from build123d import *

# Parameters (mm, degrees)
BOSS_EXTRUDE1_OUTLINE_R = 16
BOSS_EXTRUDE1_DEPTH     = 10
SKETCH2_R               = 3.025
CUT_EXTRUDE1_DEPTH      = 25.738633754
CUT_EXTRUDE2_START      = -7.5
SKETCH3_R               = 16
SKETCH3_R_2             = 6.025
CUT_EXTRUDE2_DEPTH      = 7.5
SKETCH4_R               = 1.25
CUT_EXTRUDE3_DEPTH      = 10
CUT_EXTRUDE4_DEPTH      = 10
BOSS_EXTRUDE2_START     = -2.5
BOSS_EXTRUDE2_DEPTH     = 2.5
BOSS_EXTRUDE3_START     = 2.5
SKETCH9_R               = 3.025
BOSS_EXTRUDE3_DEPTH     = 2.5
SKETCH10_R              = 5.025
CUT_EXTRUDE5_DEPTH      = 2


# Read off the part's stored shape, not the designer's step: Boss-Extrude1, Boss-Extrude2
with BuildPart() as part:
    # Boss-Extrude1 outline → Boss-Extrude1 (new body)
    with BuildSketch(Plane(origin=(0, 0, 0), x_dir=(1, 0, 0), z_dir=(0, 1, 0))):
        Circle(BOSS_EXTRUDE1_OUTLINE_R)
    extrude(amount=BOSS_EXTRUDE1_DEPTH)

    # Sketch2 → Cut-Extrude1 (cut, through all)
    with BuildSketch(Plane(origin=(0, 10, 0), x_dir=(1, 0, 0), z_dir=(0, 1, 0))):
        with Locations(Location((0, 0, 0), (0, 0, 270))):
            Circle(SKETCH2_R)
    extrude(amount=-CUT_EXTRUDE1_DEPTH, mode=Mode.SUBTRACT)

    # Sketch3 → Cut-Extrude2 (cut)
    with BuildSketch(Plane(origin=(0, 10, 0), x_dir=(1, 0, 0), z_dir=(0, 1, 0)).offset(CUT_EXTRUDE2_START)):
        with Locations(Location((0, 0, 0), (0, 0, 270))):
            Circle(SKETCH3_R)
        with Locations(Location((0, 0, 0), (0, 0, 270))):
            Circle(SKETCH3_R_2, mode=Mode.SUBTRACT)
    extrude(amount=CUT_EXTRUDE2_DEPTH, mode=Mode.SUBTRACT)

    # Sketch4 → Cut-Extrude3 (cut)
    with BuildSketch(Plane.XY):
        with Locations((0, 6.5)):
            Circle(SKETCH4_R)
    extrude(amount=-CUT_EXTRUDE3_DEPTH, mode=Mode.SUBTRACT)

    # Sketch5 → Cut-Extrude4 (cut)
    with BuildSketch(Plane(origin=(0, 0, 0), x_dir=(-1, 0, 0), z_dir=(0, -1, 0))):
        with BuildLine():
            Line((0.210340042, 14.04358534), (0.548392997, 8.04358534))
            ThreePointArc((0.548392997, 8.04358534), (-0.393770609, 6.988915846), (-1.448440102, 7.931079452))
            Line((-1.448440102, 7.931079452), (-1.786493057, 13.931079452))
            ThreePointArc((-1.786493057, 13.931079452), (-0.844329452, 14.985748945), (0.210340042, 14.04358534))
        make_face()
        with BuildLine():
            Line((13.931079452, 1.786493057), (7.931079452, 1.448440102))
            ThreePointArc((7.931079452, 1.448440102), (6.988915846, 0.393770609), (8.04358534, -0.548392997))
            Line((8.04358534, -0.548392997), (14.04358534, -0.210340042))
            ThreePointArc((14.04358534, -0.210340042), (14.985748945, 0.844329452), (13.931079452, 1.786493057))
        make_face()
        with BuildLine():
            Line((1.786493057, -13.931079452), (1.448440102, -7.931079452))
            ThreePointArc((1.448440102, -7.931079452), (0.393770609, -6.988915846), (-0.548392997, -8.04358534))
            Line((-0.548392997, -8.04358534), (-0.210340042, -14.04358534))
            ThreePointArc((-0.210340042, -14.04358534), (0.844329452, -14.985748945), (1.786493057, -13.931079452))
        make_face()
        with BuildLine():
            Line((-13.931079452, -1.786493057), (-7.931079452, -1.448440102))
            ThreePointArc((-7.931079452, -1.448440102), (-6.988915846, -0.393770609), (-8.04358534, 0.548392997))
            Line((-8.04358534, 0.548392997), (-14.04358534, 0.210340042))
            ThreePointArc((-14.04358534, 0.210340042), (-14.985748945, -0.844329452), (-13.931079452, -1.786493057))
        make_face()
    extrude(amount=-CUT_EXTRUDE4_DEPTH, mode=Mode.SUBTRACT)

    # Boss-Extrude2 outline → Boss-Extrude2 (add)
    with BuildSketch(Plane.XZ.offset(BOSS_EXTRUDE2_START)):
        with BuildLine():
            Line((-4.70856839, 45.405985014), (-4.262641267, 37.491359232))
            add(Edge.make_bspline(
                [(-4.262641267, 37.491359232), (-4.273296685, 36.107939283), (-4.30106716, 34.802769075), (-4.343751974, 33.571480974)],
                knots=[0.099174475, 0.099174475, 0.099174475, 0.099174475, 0.155965257, 0.155965257, 0.155965257, 0.155965257], degree=3))
            add(Edge.make_bspline(
                [(-4.343751974, 33.571480974), (-4.363830382, 16.861397245), (-8.211036006, 13.732402838)],
                knots=[0.224223151, 0.224223151, 0.224223151, 0.938226666, 0.938226666, 0.938226666], degree=2))
            ThreePointArc((-8.211036006, 13.732402838), (-0.370996908, 15.995698212), (7.565543006, 14.098317596))
            add(Edge.make_bspline(
                [(0.283514356, 45.687249745), (1.800888573, 18.755833196), (6.7530796, 14.602380887), (7.565543006, 14.098317596)],
                knots=[0, 0, 0, 0, 0.916762244, 0.916762244, 0.916762244, 0.916762244], degree=3))
            ThreePointArc((0.283514356, 45.687249745), (-2.353159383, 48.042658753), (-4.70856839, 45.405985014))
        make_face()
    extrude(amount=BOSS_EXTRUDE2_DEPTH)

    # Sketch9 → Boss-Extrude3 (add)
    with BuildSketch(Plane.XZ.offset(BOSS_EXTRUDE3_START)):
        with BuildLine():
            Line((-4.70856839, 45.405985014), (-4.262641267, 37.491359232))
            add(Edge.make_bspline(
                [(-4.262641267, 37.491359232), (-4.273296685, 36.107939283), (-4.30106716, 34.802769075), (-4.343751974, 33.571480974)],
                knots=[0.099174475, 0.099174475, 0.099174475, 0.099174475, 0.155965257, 0.155965257, 0.155965257, 0.155965257], degree=3))
            add(Edge.make_bspline(
                [(-4.343751974, 33.571480974), (-4.363830382, 16.861397245), (-8.211036006, 13.732402838)],
                knots=[0, 0, 0, 1, 1, 1], degree=2))
            ThreePointArc((-8.211036006, 13.732402838), (0.370996908, -15.995698212), (7.565543006, 14.098317596))
            add(Edge.make_bspline(
                [(7.565543006, 14.098317596), (6.7530796, 14.602380887), (1.800888573, 18.755833196), (0.283514356, 45.687249745)],
                knots=[0, 0, 0, 0, 0.916762244, 0.916762244, 0.916762244, 0.916762244], degree=3))
            ThreePointArc((0.283514356, 45.687249745), (-2.353159383, 48.042658753), (-4.70856839, 45.405985014))
        make_face()
        with Locations(Location((0, 0, 0), (0, 0, 90))):
            Circle(SKETCH9_R, mode=Mode.SUBTRACT)
        with BuildLine():
            Line((-1.786493057, 13.931079452), (-1.448440102, 7.931079452))
            ThreePointArc((-1.448440102, 7.931079452), (-0.393770609, 6.988915846), (0.548392997, 8.04358534))
            Line((0.548392997, 8.04358534), (0.210340042, 14.04358534))
            ThreePointArc((0.210340042, 14.04358534), (-0.844329452, 14.985748945), (-1.786493057, 13.931079452))
        make_face(mode=Mode.SUBTRACT)
        with BuildLine():
            Line((-13.931079452, -1.786493057), (-7.931079452, -1.448440102))
            ThreePointArc((-7.931079452, -1.448440102), (-6.988915846, -0.393770609), (-8.04358534, 0.548392997))
            Line((-8.04358534, 0.548392997), (-14.04358534, 0.210340042))
            ThreePointArc((-14.04358534, 0.210340042), (-14.985748945, -0.844329452), (-13.931079452, -1.786493057))
        make_face(mode=Mode.SUBTRACT)
        with BuildLine():
            Line((1.786493057, -13.931079452), (1.448440102, -7.931079452))
            ThreePointArc((1.448440102, -7.931079452), (0.393770609, -6.988915846), (-0.548392997, -8.04358534))
            Line((-0.548392997, -8.04358534), (-0.210340042, -14.04358534))
            ThreePointArc((-0.210340042, -14.04358534), (0.844329452, -14.985748945), (1.786493057, -13.931079452))
        make_face(mode=Mode.SUBTRACT)
        with BuildLine():
            Line((13.931079452, 1.786493057), (7.931079452, 1.448440102))
            ThreePointArc((7.931079452, 1.448440102), (6.988915846, 0.393770609), (8.04358534, -0.548392997))
            Line((8.04358534, -0.548392997), (14.04358534, -0.210340042))
            ThreePointArc((14.04358534, -0.210340042), (14.985748945, 0.844329452), (13.931079452, 1.786493057))
        make_face(mode=Mode.SUBTRACT)
    extrude(amount=-BOSS_EXTRUDE3_DEPTH)

    # Sketch10 → Cut-Extrude5 (cut)
    with BuildSketch(Plane.XZ.offset(2.5)):
        with Locations(Location((0, 0, 0), (0, 0, 270))):
            Circle(SKETCH10_R)
    extrude(amount=-CUT_EXTRUDE5_DEPTH, mode=Mode.SUBTRACT)


solid = part.part
Here's how the part is built. I have some questions about the finished solid (model axes, mm). A direction names the side the tool comes from. Round coordinates to 2 decimals unless told otherwise and drop trailing zeros. Write each loop counter-clockwise with the first axis right and the second up, starting at its lowest first coordinate (ties: lowest second). Pieces come first, ordered by that corner, then holes.
1. Suppose I cut it at B-B (y = 3.75). List the corners of the cut face in (x, z) for me (3 decimals).
2. Suppose I cut it at A-A (x = -12). List the corners of the cut face in (y, z) for me, and give its area (3 significant figures).
3. If we mould it in two halves opening along Y, with no side actions, what happens to faces 1 (the flat face through (10.97, -0.04, 1.62)), 2 (the flat face through (-3, 2.5, 8)), 3 (the flat face through (0.1, -0.5, -3.3)), 4 (the cylindrical face through (-1.25, 6.55, -4.37))? For each: released by +Y, released by -Y, zero draft, split by the parting line, or undercut.
4. Suppose I cut it at C-C (y = -1.5). State how many separate pieces and enclosed holes the cut face has, and give its area (3 significant figures).
5. I need wall thicknesses on L1, parallel to X at y = 3.75, z = 0 (3 decimals); L2, parallel to X at y = -1.55, z = 0 (3 decimals); L3, parallel to X at y = 6.5, z = -3.85. Which ranges of each line are inside material? Lowest first, please.
6. Will these pins go through, and if not, where does the flat tip stop? pin 1 Ø9.5 at (x, z) = (4.5, 30.5) entering from +Y; pin 2 Ø2 at (x, y) = (0, 6.5) entering from +Z (3 decimals); pin 3 Ø1 at (x, y) = (-10.5, 1.5) entering from +Z.
7. For faces 5 (the cylindrical face through (0.416, -0.035, -6.988)), 6 (the cylindrical face through (1.81, 6.198, 5.747)), 7 (the flat face through (-4, -2.5, 9)), 8 (the cylindrical face through (0.22, -1.51, 5.02)), which set-ups out of +Z, -Z, +X, -X, +Y, -Y let a thin tool reach every point of the face, with its end or its side?
Answer sheet:
1. outline: circle Ø12.05 at (0, 0); hole circle Ø6.05 at (0, 0)
2. outline: (-2.5, -10.58) - (2.5, -10.58) - (2.5, -1.68) - (-2.5, -1.68) - close; (-2.5, 0.33) - (2.5, 0.33) - (2.5, 10.58) - (-2.5, 10.58) - close
2. area: 95.8 mm2
3. face 1: zero draft
3. face 2: released by +Y
3. face 3: released by -Y
3. face 4: undercut
4. separate pieces: 1
4. enclosed holes: 5
4. area: 884 mm2
5. L1: x = -6.025 to -3.025, 3.025 to 6.025
5. L2: x = -16 to -14.603, -7.094 to -5.025, 5.025 to 7.094, 14.603 to 16
5. L3: x = -4.63 to -1.25, 1.25 to 4.63
6. pin 1: stops at y = 2.5
6. pin 2: stops at z = 6.025
6. pin 3: stops at z = 12.49
7. face 5: +Y, -Y
7. face 6: +Y
7. face 7: +Z, -Z, +X, -X, -Y
7. face 8: -Y
